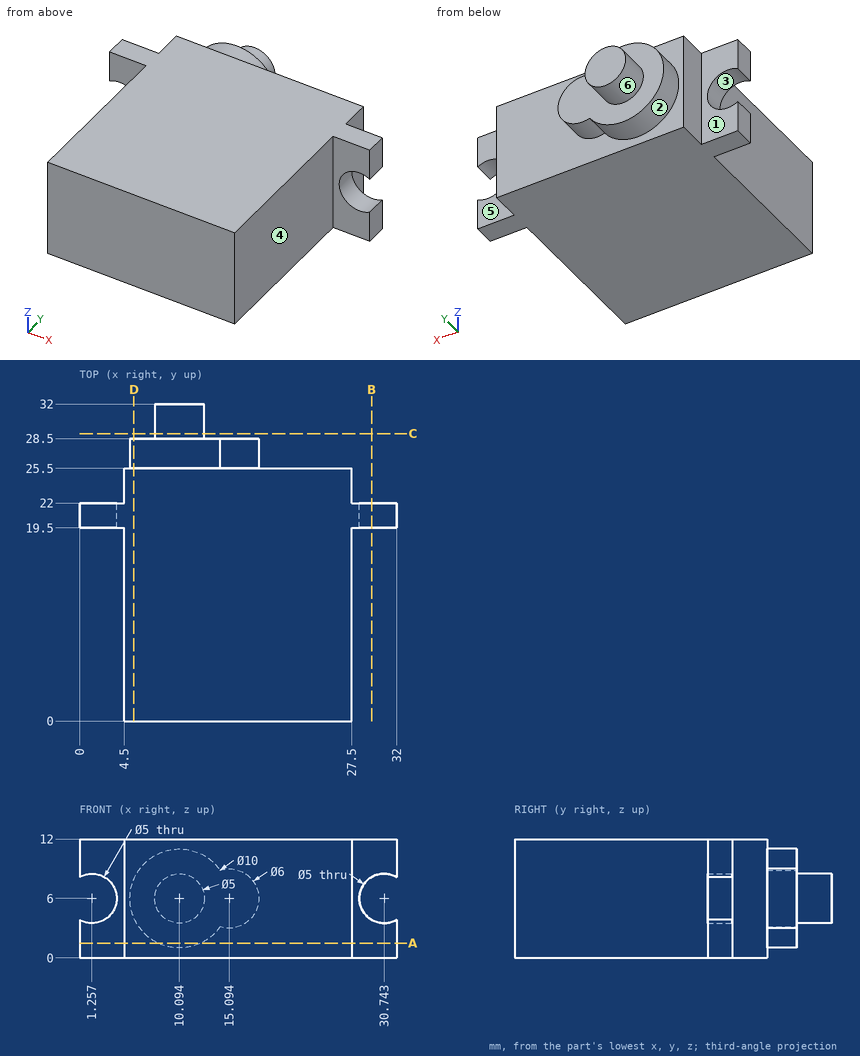
Verification items for this drawing (mm, ordinates from the low corner). A direction names the side the tool comes from. Coordinates: 2 decimals unless noted, no trailing zeros. Write each loop counter-clockwise with the first axis right and the second up, starting at its lowest first coordinate (ties: lowest second). Pieces come first, ordered by that corner, then holes. Notation, with made-up numbers: M 66.25,10.25 L 98.25,10.25 A30 cw 98.25,38.25 Z; hole C 12,59.25 d6. An arc over 180 degrees is marked long. One line per item, written item: value. Start each with the question number.
(1) Release check for a two-part mould opening along Z. For the marked faces 1, 2 and 3 record: released by +Z, released by -Z, zero draft, split by the parting line, or undercut.
(2) Tool access check on the marked faces 4, 5 and 6. Record the directions out of +Z, -Z, +X, -X, +Y, -Y that give a thin tool (end or side, any length) a straight path to the whole face; none if there is none.
(3) Sectioned sample at B-B, the plane x = 29.5. Enter the section's corners in (y, z).
(4) Scan lines: line 1 along Y through (x, z) = (19, 1); line 2 along X through (y, z) = (2, 1.25); line 3 along X through (y, z) = (21.05, 6). Record each from-to range of solid material in increasing order. Write a range as [from, to].
(5) Depth check by flat-ended pin: pin 1 (2 mm diameter, centred on y = 25, z = 4.5, fed in from +X); pin 2 (5 mm diameter, centred on x = 1.5, z = 5, fed in from -Y); pin 3 (1.5 mm diameter, centred on x = 12, z = 2.5, fed in from +Y). Enter the tip coordinate at first touch or a pass-through.
(6) Sectioned sample at D-D, the plane x = 5.5. Enter the section's corners in (y, z), and give its area (3 significant figures).
(7) Sectioned sample at C-C, the plane y = 29. Enter the section's corners in (x, z), and give its area (3 significant figures).
(8) Sectioned sample at A-A, the plane z = 1.5. Enter the section's corners in (x, y), and give its area (3 significant figures).
Filled sheet:
1. face 1: zero draft
1. face 2: split by the parting line
1. face 3: undercut
2. face 4: +Z, -Z, +X, -Y
2. face 5: +Z, -Z, +X, +Y
2. face 6: +Y
3. outline: M 19.5,0 L 22,0 L 22,3.83 L 19.5,3.83 Z; M 19.5,8.17 L 22,8.17 L 22,12 L 19.5,12 Z
4. line 1: [0, 25.5]
4. line 2: [4.5, 27.5]
4. line 3: [3.76, 28.24]
5. pin 1: x = 27.5
5. pin 2: y = 19.5
5. pin 3: y = 28.5
6. outline: M 0,0 L 25.5,0 L 25.5,4.03 L 28.5,4.03 L 28.5,7.97 L 25.5,7.97 L 25.5,12 L 0,12 Z
6. area: 318 mm²
7. outline: C 10.09,6 d5
7. area: 19.6 mm²
8. outline: M 0,19.5 L 4.5,19.5 L 4.5,0 L 27.5,0 L 27.5,19.5 L 32,19.5 L 32,22 L 27.5,22 L 27.5,25.5 L 12.27,25.5 L 12.27,28.5 L 7.91,28.5 L 7.91,25.5 L 4.5,25.5 L 4.5,22 L 0,22 Z
8. area: 622 mm²
